```python
from build123d import *

# Parameters (mm, degrees)
SKETCH_1_W           = 40
SKETCH_1_H           = 29
EXTRUDE_1_DEPTH      = 3
CUT_EXTRUDE_1_DEPTH  = 3
SKETCH_3_W           = 40
SKETCH_3_H           = 3
EXTRUDE_2_DEPTH      = 10
SKETCH_4_W           = 40
SKETCH_4_H           = 3
EXTRUDE_3_DEPTH      = 10
SKETCH_6_W           = 3
SKETCH_6_H           = 49
EXTRUDE_5_DEPTH      = 42
SKETCH_8_W           = 3
SKETCH_8_H           = 49
EXTRUDE_6_DEPTH      = 2
SKETCH_9_W           = 3
SKETCH_9_H           = 49
EXTRUDE_7_DEPTH      = 2
SKETCH_10_W          = 86
SKETCH_10_H          = 3
EXTRUDE_8_DEPTH      = 10
SKETCH_11_W          = 86
SKETCH_11_H          = 3
EXTRUDE_9_DEPTH      = 10
SKETCH_14_W          = 3
SKETCH_14_H          = 69
CUT_EXTRUDE_5_DEPTH  = 43
SKETCH_17_W          = 43
SKETCH_17_H          = 3
EXTRUDE_10_DEPTH     = 20
SKETCH_20_W          = 43
SKETCH_20_H          = 3
EXTRUDE_11_DEPTH     = 10
SKETCH_21_W          = 43
SKETCH_21_H          = 3
CUT_EXTRUDE_7_DEPTH  = 20
SKETCH_24_R          = 2.2
CUT_EXTRUDE_8_DEPTH  = 30
SKETCH_26_R          = 1.6
CUT_EXTRUDE_9_DEPTH  = 10
SKETCH_27_W          = 3
SKETCH_27_H          = 79
CUT_EXTRUDE_10_DEPTH = 8
SKETCH_28_W          = 35
SKETCH_28_H          = 3
CUT_EXTRUDE_11_DEPTH = 15
CUT_EXTRUDE_13_DEPTH = 10
M4X0_7_3_D           = 3.3


with BuildPart() as part:
    # ｽｹｯﾁ1 → ﾎﾞｽ - 押し出し1 (new body)
    with BuildSketch(Plane.XY):
        Rectangle(SKETCH_1_W, SKETCH_1_H)
    extrude(amount=EXTRUDE_1_DEPTH)

    # ｽｹｯﾁ2 → ｶｯﾄ - 押し出し1 (cut)
    with BuildSketch(Plane.XY.offset(3)):
        with BuildLine():
            ThreePointArc((-14.4, 10.5), (-15.01507576, 11.98492424), (-16.5, 12.6))
            Line((-16.5, 12.6), (-16.5, 10.5))
            Line((-16.5, 10.5), (-18.6, 10.5))
            ThreePointArc((-18.6, 10.5), (-16.5, 8.4), (-14.4, 10.5))
        make_face()
        with BuildLine():
            Line((-16.5, 10.5), (-16.5, 12.6))
            ThreePointArc((-16.5, 12.6), (-17.98492424, 11.98492424), (-18.6, 10.5))
            Line((-18.6, 10.5), (-16.5, 10.5))
        make_face()
        with BuildLine():
            ThreePointArc((-18.6, -10.5), (-17.98492424, -11.98492424), (-16.5, -12.6))
            Line((-16.5, -12.6), (-16.5, -10.5))
            Line((-16.5, -10.5), (-18.6, -10.5))
        make_face()
        with BuildLine():
            Line((-16.5, -10.5), (-16.5, -12.6))
            ThreePointArc((-16.5, -12.6), (-15.01507576, -11.98492424), (-14.4, -10.5))
            ThreePointArc((-14.4, -10.5), (-16.5, -8.4), (-18.6, -10.5))
            Line((-18.6, -10.5), (-16.5, -10.5))
        make_face()
        with BuildLine():
            ThreePointArc((18.6, -10.5), (15.01507576, -9.01507576), (16.5, -12.6))
            Line((16.5, -12.6), (16.5, -10.5))
            Line((16.5, -10.5), (18.6, -10.5))
        make_face()
        with BuildLine():
            Line((16.5, -10.5), (16.5, -12.6))
            ThreePointArc((16.5, -12.6), (17.98492424, -11.98492424), (18.6, -10.5))
            Line((18.6, -10.5), (16.5, -10.5))
        make_face()
        with BuildLine():
            ThreePointArc((18.6, 10.5), (17.98492424, 11.98492424), (16.5, 12.6))
            Line((16.5, 12.6), (16.5, 10.5))
            Line((16.5, 10.5), (18.6, 10.5))
        make_face()
        with BuildLine():
            Line((16.5, 10.5), (16.5, 12.6))
            ThreePointArc((16.5, 12.6), (15.01507576, 9.01507576), (18.6, 10.5))
            Line((18.6, 10.5), (16.5, 10.5))
        make_face()
    extrude(amount=-CUT_EXTRUDE_1_DEPTH, mode=Mode.SUBTRACT)

    # ｽｹｯﾁ3 → ﾎﾞｽ - 押し出し2 (add)
    with BuildSketch(Plane.XZ.offset(14.5)):
        with Locations((0, 1.5)):
            Rectangle(SKETCH_3_W, SKETCH_3_H)
    extrude(amount=EXTRUDE_2_DEPTH)

    # ｽｹｯﾁ4 → ﾎﾞｽ - 押し出し3 (add)
    with BuildSketch(Plane(origin=(0, 14.5, 0), x_dir=(1, 0, 0), z_dir=(0, 1, 0))):
        with Locations((0, -1.5)):
            Rectangle(SKETCH_4_W, SKETCH_4_H)
    extrude(amount=EXTRUDE_3_DEPTH)

    # ｽｹｯﾁ6 → ﾎﾞｽ - 押し出し5 (add)
    with BuildSketch(Plane(origin=(20, 0, 0), x_dir=(0, 0, -1), z_dir=(1, 0, 0))):
        with Locations((-1.5, 0)):
            Rectangle(SKETCH_6_W, SKETCH_6_H)
    extrude(amount=EXTRUDE_5_DEPTH)

    # ｽｹｯﾁ8 → ﾎﾞｽ - 押し出し6 (add)
    with BuildSketch(Plane.ZY.offset(20)):
        with Locations((1.5, 0)):
            Rectangle(SKETCH_8_W, SKETCH_8_H)
    extrude(amount=EXTRUDE_6_DEPTH)

    # ｽｹｯﾁ9 → ﾎﾞｽ - 押し出し7 (add)
    with BuildSketch(Plane(origin=(62, 0, 0), x_dir=(0, 0, -1), z_dir=(1, 0, 0))):
        with Locations((-1.5, 0)):
            Rectangle(SKETCH_9_W, SKETCH_9_H)
    extrude(amount=EXTRUDE_7_DEPTH)

    # ｽｹｯﾁ10 → ﾎﾞｽ - 押し出し8 (add)
    with BuildSketch(Plane.XZ.offset(24.5)):
        with Locations((21, 1.5)):
            Rectangle(SKETCH_10_W, SKETCH_10_H)
    extrude(amount=EXTRUDE_8_DEPTH)

    # ｽｹｯﾁ11 → ﾎﾞｽ - 押し出し9 (add)
    with BuildSketch(Plane(origin=(0, 24.5, 0), x_dir=(1, 0, 0), z_dir=(0, 1, 0))):
        with Locations((21, -1.5)):
            Rectangle(SKETCH_11_W, SKETCH_11_H)
    extrude(amount=EXTRUDE_9_DEPTH)

    # ｽｹｯﾁ14 → ｶｯﾄ - 押し出し5 (cut)
    with BuildSketch(Plane.ZY.offset(22)):
        with Locations((1.5, 0)):
            Rectangle(SKETCH_14_W, SKETCH_14_H)
    extrude(amount=-CUT_EXTRUDE_5_DEPTH, mode=Mode.SUBTRACT)

    # ｽｹｯﾁ17 → ﾎﾞｽ - 押し出し10 (add)
    with BuildSketch(Plane.XZ.offset(34.5)):
        with Locations((42.5, 1.5)):
            Rectangle(SKETCH_17_W, SKETCH_17_H)
    extrude(amount=EXTRUDE_10_DEPTH)

    # ｽｹｯﾁ20 → ﾎﾞｽ - 押し出し11 (add)
    with BuildSketch(Plane.XZ.offset(54.5)):
        with Locations((42.5, 1.5)):
            Rectangle(SKETCH_20_W, SKETCH_20_H)
    extrude(amount=EXTRUDE_11_DEPTH)

    # ｽｹｯﾁ21 → ｶｯﾄ - 押し出し7 (cut)
    with BuildSketch(Plane.XZ.offset(64.5)):
        with Locations((42.5, 1.5)):
            Rectangle(SKETCH_21_W, SKETCH_21_H)
    extrude(amount=-CUT_EXTRUDE_7_DEPTH, mode=Mode.SUBTRACT)

    # ｽｹｯﾁ24 → ｶｯﾄ - 押し出し8 (cut)
    with BuildSketch(Plane(origin=(0, 0, 0), x_dir=(-1, 0, 0), z_dir=(0, 0, -1))):
        with Locations((-36.27, 14.5)):
            Circle(SKETCH_24_R)
        with Locations((-57, 14.5)):
            Circle(SKETCH_24_R)
    extrude(amount=-CUT_EXTRUDE_8_DEPTH, mode=Mode.SUBTRACT)

    # ｽｹｯﾁ26 → ｶｯﾄ - 押し出し9 (cut)
    with BuildSketch(Plane(origin=(0, 0, 0), x_dir=(-1, 0, 0), z_dir=(0, 0, -1))):
        with Locations((-36.11, -7.5)):
            Circle(SKETCH_26_R)
    extrude(amount=-CUT_EXTRUDE_9_DEPTH, mode=Mode.SUBTRACT)

    # ｽｹｯﾁ27 → ｶｯﾄ - 押し出し10 (cut)
    with BuildSketch(Plane.ZY.offset(-21)):
        with Locations((1.5, -5)):
            Rectangle(SKETCH_27_W, SKETCH_27_H)
    extrude(amount=-CUT_EXTRUDE_10_DEPTH, mode=Mode.SUBTRACT)

    # ｽｹｯﾁ28 → ｶｯﾄ - 押し出し11 (cut)
    with BuildSketch(Plane(origin=(0, 34.5, 0), x_dir=(1, 0, 0), z_dir=(0, 1, 0))):
        with Locations((46.5, -1.5)):
            Rectangle(SKETCH_28_W, SKETCH_28_H)
    extrude(amount=-CUT_EXTRUDE_11_DEPTH, mode=Mode.SUBTRACT)

    # ｽｹｯﾁ33 → ｶｯﾄ - 押し出し13 (cut)
    with BuildSketch(Plane(origin=(0, 0, 0), x_dir=(-1, 0, 0), z_dir=(0, 0, -1))):
        with BuildLine():
            ThreePointArc((-35, -34.5), (-36.707106781, -33.792893219), (-36, -35.5))
            Line((-36, -35.5), (-36, -34.5))
            Line((-36, -34.5), (-35, -34.5))
        make_face()
        with BuildLine():
            Line((-36, -34.5), (-36, -35.5))
            ThreePointArc((-36, -35.5), (-35.292893219, -35.207106781), (-35, -34.5))
            Line((-35, -34.5), (-36, -34.5))
        make_face()
        with BuildLine():
            ThreePointArc((-58, -34.5), (-57.707106781, -35.207106781), (-57, -35.5))
            Line((-57, -35.5), (-57, -34.5))
            Line((-57, -34.5), (-58, -34.5))
        make_face()
        with BuildLine():
            Line((-57, -34.5), (-57, -35.5))
            ThreePointArc((-57, -35.5), (-56.292893219, -35.207106781), (-56, -34.5))
            ThreePointArc((-56, -34.5), (-57, -33.5), (-58, -34.5))
            Line((-58, -34.5), (-57, -34.5))
        make_face()
    extrude(amount=-CUT_EXTRUDE_13_DEPTH, mode=Mode.SUBTRACT)

    # M4x0.7 ねじ穴3 (through all)
    with Locations(Plane(origin=(36, -34.5, 0), x_dir=(-1, 0, 0), z_dir=(0, 0, -1))):
        with Locations((0, 0), (-21, 0)):
            Hole(M4X0_7_3_D / 2)


solid = part.part
```
Can you work these out from the model? Positions are in its coordinate system, mm. Coordinates: 2 decimals unless noted, no trailing zeros. Loops run counter-clockwise (first coordinate to the right, second up) from the corner with the lowest first, then second, coordinate; pieces in that order, holes last. Notation, with made-up numbers: (25.5, -7.5) -> (69.5, -7.5) arc R31 cw to (69.5, 24.5) -> close; hole circle Ø8 at (-33.75, 12.25). An arc over 180 degrees is marked (long way). Put each result on its own line as item: value. Start each with the question number.
Q1. I want a section at D-D (y = -7.5). Write out the boundary of the cut face in (x, z), plus the area to 3 significant figures.
Q2. Thinking about a two-plate mould opening in Y: for faces 1 (the face through (46, -44.5, 2)), 2 (the face through (46, 19.5, 1)), 3 (the face through (37.71, -7.43, 1.48)), which applies, pulls with the +Y half, pulls with the -Y half, needs draft (parallel to the pull), parting line crosses it, or undercut?
Q3. I want a section at B-B (z = 0.65). Write out the boundary of the cut face in (x, y).
Q4. I want a section at A-A (x = 57). Write out the boundary of the cut face in (y, z).
Q5. I want a section at C-C (y = -34.5). Write out the boundary of the cut face in (x, z).
Q6. If I drill on line 1 (Y direction, x = 57, z = 1.8); line 2 (Y direction, x = 36.27, z = 1.35); line 3 (X direction, y = -8.5, z = 0.75), over which ranges is the centre line in solid material (lowest first)? Write a range as [from, to].
Taken from the geometry:
1. outline: (29, 0) -> (34.51, 0) -> (34.51, 3) -> (29, 3) -> close; (37.71, 0) -> (64, 0) -> (64, 3) -> (37.71, 3) -> close
1. area: 95.4 mm2
2. face 1: pulls with the -Y half
2. face 2: pulls with the +Y half
2. face 3: undercut
3. outline: (29, -44.5) -> (64, -44.5) -> (64, 19.5) -> (29, 19.5) -> close; hole circle Ø4.4 at (36.27, 14.5); hole circle Ø3.3 at (36, -34.5); hole circle Ø3.2 at (36.11, -7.5); hole circle Ø4.4 at (57, 14.5); hole circle Ø3.3 at (57, -34.5)
4. outline: (-44.5, 0) -> (-36.15, 0) -> (-36.15, 3) -> (-44.5, 3) -> close; (-32.85, 0) -> (12.3, 0) -> (12.3, 3) -> (-32.85, 3) -> close; (16.7, 0) -> (19.5, 0) -> (19.5, 3) -> (16.7, 3) -> close
5. outline: (29, 0) -> (34.35, 0) -> (34.35, 3) -> (29, 3) -> close; (37.65, 0) -> (55.35, 0) -> (55.35, 3) -> (37.65, 3) -> close; (58.65, 0) -> (64, 0) -> (64, 3) -> (58.65, 3) -> close
6. line 1: y = [-44.5, -36.15], [-32.85, 12.3], [16.7, 19.5]
6. line 2: y = [-44.5, -36.13], [-32.87, -9.09], [-5.91, 12.3], [16.7, 19.5]
6. line 3: x = [29, 34.86], [37.36, 64]
